Could you check a few things on this model? Use its own coordinates, in mm. Face numbers are marked on the shaded views. A direction names the side the tool comes from. Round coordinates to 2 decimals unless told otherwise and drop trailing zeros. Write each loop counter-clockwise with the first axis right and the second up, starting at its lowest first coordinate (ties: lowest second). Pieces come first, ordered by that corner, then holes. Notation, with made-up numbers: (-15.75, 7.25) -> (27.25, 7.25) arc R34 ccw to (27.25, 40.25) -> close; hole circle Ø6 at (32, 53). An arc over 180 degrees is marked (long way). Return JSON: item names as keys, results as strings.
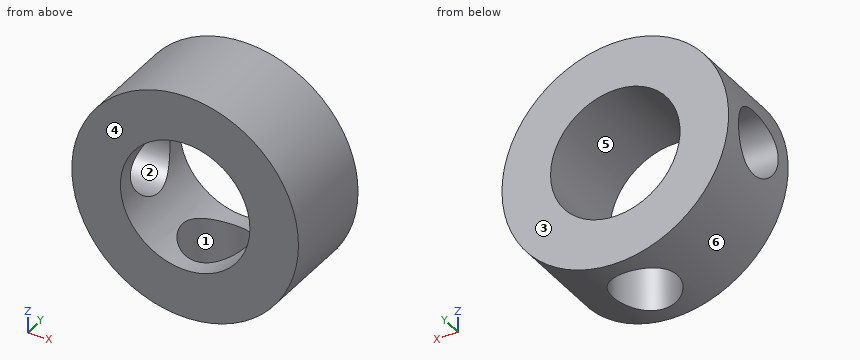
from build123d import *

# Parameters (mm, degrees)
SKETCH_1_R          = 7
SKETCH_1_R_2        = 4
EXTRUDE_1_DEPTH     = 6
SKETCH_2_R          = 2
CUT_EXTRUDE_1_DEPTH = 10
SKETCH_3_R          = 2
CUT_EXTRUDE_2_DEPTH = 10


with BuildPart() as part:
    # 草图1 → 凸台-拉伸1 (new body)
    with BuildSketch(Plane(origin=(0, 0, 0), x_dir=(1, 0, 0), z_dir=(0, 1, 0))):
        Circle(SKETCH_1_R)
        Circle(SKETCH_1_R_2, mode=Mode.SUBTRACT)
    extrude(amount=EXTRUDE_1_DEPTH)

    # 草图2 → 切除-拉伸1 (cut)
    with BuildSketch(Plane(origin=(0, 0, 0), x_dir=(0, 0, -1), z_dir=(1, 0, 0))):
        with Locations((0, 3)):
            Circle(SKETCH_2_R)
    extrude(amount=-CUT_EXTRUDE_1_DEPTH, mode=Mode.SUBTRACT)

    # 草图3 → 切除-拉伸2 (cut)
    with BuildSketch(Plane.XY):
        with Locations((0, 3)):
            Circle(SKETCH_3_R)
    extrude(amount=-CUT_EXTRUDE_2_DEPTH, mode=Mode.SUBTRACT)


solid = part.part
1) I want a section at A-A, the plane x = 0. Please give me the cut outline in (y, z).
Return value:
{"outline": "(0, -7) -> (1, -7) -> (1, -4) -> (0, -4) -> close; (0, 4) -> (6, 4) -> (6, 7) -> (0, 7) -> close; (5, -7) -> (6, -7) -> (6, -4) -> (5, -4) -> close"}
2) I want a section at B-B, the plane z = 0. Please give me the cut outline in (x, y).
Return value:
{"outline": "(-7, 0) -> (-4, 0) -> (-4, 1) -> (-7, 1) -> close; (-7, 5) -> (-4, 5) -> (-4, 6) -> (-7, 6) -> close; (4, 0) -> (7, 0) -> (7, 6) -> (4, 6) -> close"}
3) Will these pins go through, and if not, where does the flat tip stop? pin 1 Ø6.5 at (x, z) = (0, 0) entering from +Y; pin 2 Ø2 at (x, y) = (4.5, 4) entering from +Z; pin 3 Ø3.5 at (y, z) = (3, 0) entering from -X.
Return value:
{"pin 1": "through", "pin 2": "z = 6.06", "pin 3": "x = 3.6"}
4) If I drill on probe 1 along Y at (x, z) = (-4.55, 0); probe 2 along Z at (x, y) = (-2.25, 5.5); probe 3 along X at (y, z) = (3, -5.05), over which ranges is the centre line in solid material (lowest first)? Write a range as [from, to].
Return value:
{"probe 1": "[0, 1], [5, 6]", "probe 2": "[-6.63, -3.31], [3.31, 6.63]", "probe 3": "[-4.85, -2], [2, 4.85]"}
5) I want a section at D-D, the plane z = -2.25. Please give me the cut outline in (x, y).
Return value:
{"outline": "(-6.63, 0) -> (-3.31, 0) -> (-3.31, 6) -> (-6.63, 6) -> close; (3.31, 0) -> (6.63, 0) -> (6.63, 6) -> (3.31, 6) -> close"}
6) Thinking about a two-plate mould opening in Z: for the marked faces 4, 5 and 6, which applies, pulls with the +Z half, pulls with the -Z half, needs draft (parallel to the pull), parting line crosses it, or undercut?
Return value:
{"face 4": "needs draft", "face 5": "undercut", "face 6": "parting line crosses it"}
7) For the marked faces 1, 2 and 3, which set-ups out of +Z, -Z, +X, -X, +Y, -Y let a thin tool reach every point of the face, with its end or its side?
Return value:
{"face 1": "-Z", "face 2": "-X", "face 3": "+Z, -Z, +X, -X, +Y"}
8) I want a section at C-C, the plane y = 3. Please give me the cut outline in (x, z).
Return value:
{"outline": "(-6.71, -2) arc R7 ccw to (-2, -6.71) -> (-2, -3.46) arc R4 cw to (-3.46, -2) -> close; (-6.71, 2) -> (-3.46, 2) arc R4 cw (long way) to (2, -3.46) -> (2, -6.71) arc R7 ccw (long way) to start"}
